Source: CAD feature listing. Evaluate the final solid. Frame: model axes, mm. Round coordinates to 2 decimals unless told otherwise and drop trailing zeros. Loops run counter-clockwise (first coordinate to the right, second up) from the corner with the lowest first, then second, coordinate; pieces in that order, holes last. Notation, with made-up numbers: (-31.5, 10.5) -> (8.5, 10.5) arc R25 ccw to (8.5, 45.5) -> close; hole circle Ø5 at (-7.5, 2). An arc over 180 degrees is marked (long way). Write item = value, one per line.
from build123d import *

# Parameters (mm, degrees)
SZKIC1_W                    = 62.3
SZKIC1_H                    = 42.9
DODANIE_WYCI_GNI_CIE1_DEPTH = 1
SZKIC5_W                    = 6
SZKIC5_H                    = 5.66
WYTNIJ_WYCI_GNI_CIE2_DEPTH  = 7
SZKIC6_R                    = 1.4
WYTNIJ_WYCI_GNI_CIE3_DEPTH  = 10
ZAOKR_GLENIE1_R             = 2
SFAZOWANIE1_SIZE            = 0.2


with BuildPart() as part:
    # Szkic1 → Dodanie-wyciągnięcie1 (new body)
    with BuildSketch(Plane(origin=(0, 0, 0), x_dir=(1, 0, 0), z_dir=(0, 1, 0))):
        Rectangle(SZKIC1_W, SZKIC1_H)
    extrude(amount=DODANIE_WYCI_GNI_CIE1_DEPTH)

    # Szkic5 → Wytnij-wyciągnięcie2 (cut)
    with BuildSketch(Plane(origin=(0, 1, 0), x_dir=(1, 0, 0), z_dir=(0, 1, 0))):
        with Locations((15.29, -11.08)):
            Rectangle(SZKIC5_W, SZKIC5_H)
    extrude(amount=-WYTNIJ_WYCI_GNI_CIE2_DEPTH, mode=Mode.SUBTRACT)

    # Szkic6 → Wytnij-wyciągnięcie3 (cut)
    with BuildSketch(Plane(origin=(0, 1, 0), x_dir=(1, 0, 0), z_dir=(0, 1, 0))):
        with Locations((27.4, 18.05)):
            Circle(SZKIC6_R)
        with Locations((27.4, -18.05)):
            Circle(SZKIC6_R)
        with Locations((-27.4, -18.05)):
            Circle(SZKIC6_R)
        with Locations((-27.4, 18.05)):
            Circle(SZKIC6_R)
    extrude(amount=-WYTNIJ_WYCI_GNI_CIE3_DEPTH, mode=Mode.SUBTRACT)

    # Zaokrąglenie1
    zaokr_glenie1_edges = [part.edges().sort_by_distance(p)[0] for p in [
        (31.15, 0.5, 21.45),
        (-31.15, 0.5, 21.45),
        (-31.15, 0.5, -21.45),
        (31.15, 0.5, -21.45),
    ]]
    fillet(zaokr_glenie1_edges, radius=ZAOKR_GLENIE1_R)

    # Sfazowanie1
    sfazowanie1_edges = [part.edges().sort_by_distance(p)[0] for p in [
        (-28.8, 1, -18.05),
        (-28.8, 1, 18.05),
        (26, 1, 18.05),
        (26, 1, -18.05),
    ]]
    chamfer(sfazowanie1_edges, length=SFAZOWANIE1_SIZE)


solid = part.part
1. Section query A-A (y = 0.35). Return the cut outline in (x, z), then the cut area to 3 significant figures.
Evaluation:
outline = (-31.15, -19.45) arc R2 ccw to (-29.15, -21.45) -> (29.15, -21.45) arc R2 ccw to (31.15, -19.45) -> (31.15, 19.45) arc R2 ccw to (29.15, 21.45) -> (-29.15, 21.45) arc R2 ccw to (-31.15, 19.45) -> close; hole circle Ø2.8 at (-27.4, -18.05); hole circle Ø2.8 at (-27.4, 18.05); hole (12.29, 8.25) -> (18.29, 8.25) -> (18.29, 13.91) -> (12.29, 13.91) -> close; hole circle Ø2.8 at (27.4, -18.05); hole circle Ø2.8 at (27.4, 18.05)
area = 2,610 mm²
2. Mould query, pull axis X, two halves, no side actions, for faces 1 (the face through (30.55, 0.51, -20.88)), 2 (the face through (-30.58, 0.51, 20.85)), 3 (the face through (-26.11, 0.41, -17.51)). Classes: released by +X, released by -X, zero draft, split by the parting line, or undercut.
Evaluation:
face_1 = released by +X
face_2 = released by -X
face_3 = undercut
3. Contact query for flat-ended pins moving along their axis: pin 1 Ø3 at (x, z) = (27.4, -18.05) entering from +Y; pin 2 Ø4.5 at (x, z) = (-27.4, -18.05) entering from -Y. Output: stop coordinate, or through.
Evaluation:
pin_1 = 0.9
pin_2 = 0
4. Line query: probe 1 along Z at (x, y) = (-27.4, 0.2); probe 2 along X at (y, z) = (0.3, -18.05); probe 3 along X at (y, z) = (0.7, 11). Output: solid intervals per line, ascending. Write a range as from..to.
Evaluation:
probe_1 = -21.45..-19.45, -16.65..16.65, 19.45..21.45
probe_2 = -31.15..-28.8, -26..26, 28.8..31.15
probe_3 = -31.15..12.29, 18.29..31.15
5. Section query D-D (z = 18.05). Return the cut outline in (x, y), then the cut area to 3 significant figures.
Evaluation:
outline = (-31.15, 0) -> (-28.8, 0) -> (-28.8, 0.8) -> (-29, 1) -> (-31.15, 1) -> close; (-26, 0) -> (26, 0) -> (26, 0.8) -> (25.8, 1) -> (-25.8, 1) -> (-26, 0.8) -> close; (28.8, 0) -> (31.15, 0) -> (31.15, 1) -> (29, 1) -> (28.8, 0.8) -> close
area = 56.6 mm²
6. Section query C-C (x = -27.4). Return the cut outline in (y, z).
Evaluation:
outline = (0, -21.45) -> (1, -21.45) -> (1, -19.65) -> (0.8, -19.45) -> (0, -19.45) -> close; (0, -16.65) -> (0.8, -16.65) -> (1, -16.45) -> (1, 16.45) -> (0.8, 16.65) -> (0, 16.65) -> close; (0, 19.45) -> (0.8, 19.45) -> (1, 19.65) -> (1, 21.45) -> (0, 21.45) -> close
7. Section query B-B (z = 9.5). Return the cut outline in (x, y).
Evaluation:
outline = (-31.15, 0) -> (12.29, 0) -> (12.29, 1) -> (-31.15, 1) -> close; (18.29, 0) -> (31.15, 0) -> (31.15, 1) -> (18.29, 1) -> close
